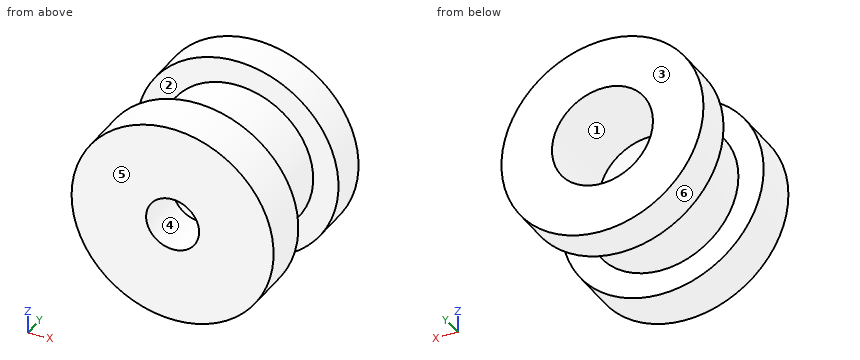
Autodesk Inventor part; units mm, degrees
ref_plane "YZ Plane" through (0, 0, 0) normal (1, 0, 0) x (0, 1, 0)
ref_plane "XZ Plane" through (0, 0, 0) normal (0, 1, 0) x (-1, 0, 0)
ref_plane "XY Plane" through (0, 0, 0) normal (0, 0, 1) x (1, 0, 0)
sketch "Sketch1" plane through (0, 0, 0) normal (0, 0, 1) x (1, 0, 0)
  line L0 (-2.1, -6.7) -> (-8, -6.7)
  line L1 (-8, -6.7) -> (-8, -3)
  line L2 (-8, -3) -> (-6, -3)
  line L3 (-6, -3) -> (-6, 3)
  line L4 (-6, 3) -> (-8, 3)
  line L5 (-8, 3) -> (-8, 6)
  line L6 (-8, 6) -> (-4, 6)
  line L7 (0, 0) -> (-16, 0) construction
  line L8 (0, -9.24) -> (0, 8.54)
  line L9 (-2.1, -6.7) -> (-2.1, -2.7)
  line L10 (-2.1, -2.7) -> (-4, -1)
  line L11 (-4, -1) -> (-4, 6)
  dimension "d1" = 8
  dimension "d2" = 3.7
  dimension "d3" = 3
  dimension "d4" = 6
  dimension "d5" = 6
  dimension "d7" = 4
  dimension "d8" = 2.1
  dimension "d9" = 7
  dimension "d11" = 4
revolve "Revolution2" add sketch "Sketch1" angle 360 about axis through (0, -10, 0) along (0, 1, 0)
properties part number "Groove_Mount_Adaptor_1_75mm"
The model under review builds one solid part; all positions refer to its coordinate system, in mm. Face numbers are marked on the shaded views. A direction names the side the tool comes from. Round coordinates to 2 decimals unless told otherwise and drop trailing zeros. Order: outer loops, then holes, each group sorted by start corner. A loop starts at its lowest first (then second) coordinate and runs counter-clockwise, first axis right, second up. Notation, with made-up numbers: (13.5, 53.25) -> (60.5, 53.25) arc R17 cw to (60.5, 64.25) -> close; hole circle Ø3 at (-21.75, 75). An arc over 180 degrees is marked (long way). One line per item, written item: value. Start each with the question number.
Q1. Take a section at C-C (y = 1.5). Write out the cut boundary in (x, z), and give its area (3 significant figures).
Q2. Clearance check with flat-ended pins moving along their axes: pin 1 Ø1 at (y, z) = (-1, -5.5) entering from -X; pin 2 Ø4 at (y, z) = (-4, -5) entering from -X; pin 3 Ø4 at (x, y) = (-2.5, -2) entering from -Z. State where each tip first meets the part, or that it passes through.
Q3. Take a section at B-B (x = 0). Write out the cut boundary in (y, z), and give its area (3 significant figures).
Q4. Wall thickness on line 1 (Z direction, x = 0, y = 1); line 2 (Z direction, x = 0, y = 3.5); line 3 (Y direction, x = -0.75, z = 6.75): over which ranges is each line inside the solid? List them lowest first.
Q5. Machinability: for the marked faces 1, 2 and 3, which of the approach directions +Z, -Z, +X, -X, +Y, -Y give a long, thin tool a straight path to every point of the face, cutting with its end or side? Answer none if there is none.
Q6. Take a section at A-A (z = 0). Write out the cut boundary in (x, y).
Q7. Mouldability with a two-part tool opening along Z and no side actions: class the marked faces 4, 5 and 6 as released by +Z, released by -Z, zero draft, split by the parting line, or undercut.
Q8. Take a section at D-D (x = -4.5). Write out the cut boundary in (y, z), and give its area (3 significant figures).
Reported:
1. outline: circle Ø12 at (0, 0); hole circle Ø8 at (0, 0)
1. area: 62.8 mm2
2. pin 1: stops at x = -3.32
2. pin 2: stops at x = -7.42
2. pin 3: stops at z = -7.96
3. outline: (-6.7, -8) -> (-3, -8) -> (-3, -6) -> (3, -6) -> (3, -8) -> (6, -8) -> (6, -4) -> (-1, -4) -> (-2.7, -2.1) -> (-6.7, -2.1) -> close; (-6.7, 2.1) -> (-2.7, 2.1) -> (-1, 4) -> (6, 4) -> (6, 8) -> (3, 8) -> (3, 6) -> (-3, 6) -> (-3, 8) -> (-6.7, 8) -> close
3. area: 96.0 mm2
4. line 1: z = -6 to -4, 4 to 6
4. line 2: z = -8 to -4, 4 to 8
4. line 3: y = -6.7 to -3, 3 to 6
5. face 1: +Y
5. face 2: none
5. face 3: +Z, -Z, +X, -X, +Y
6. outline: (-8, -6.7) -> (-2.1, -6.7) -> (-2.1, -2.7) -> (-4, -1) -> (-4, 6) -> (-8, 6) -> (-8, 3) -> (-6, 3) -> (-6, -3) -> (-8, -3) -> close; (2.1, -6.7) -> (8, -6.7) -> (8, -3) -> (6, -3) -> (6, 3) -> (8, 3) -> (8, 6) -> (4, 6) -> (4, -1) -> (2.1, -2.7) -> close
7. face 4: undercut
7. face 5: zero draft
7. face 6: split by the parting line
8. outline: (-6.7, -6.61) -> (-3, -6.61) -> (-3, -3.97) -> (3, -3.97) -> (3, -6.61) -> (6, -6.61) -> (6, 6.61) -> (3, 6.61) -> (3, 3.97) -> (-3, 3.97) -> (-3, 6.61) -> (-6.7, 6.61) -> close
8. area: 136 mm2
